```python
from build123d import *

# Parameters (mm, degrees)
F1_DEPTH = 63.5


with BuildPart() as f1:
    # F0 (on Front) → F1 (new body, symmetric)
    with BuildSketch(Plane.XZ):
        Polygon((60.325, 71.4502), (60.325, 61.5735440695), (83.1756805858, 61.5735440695), (83.1756805858, 42.8752), (111.125, 42.8752), (111.125, 71.4502), align=None)
        Polygon((22.225, 9.525), (-41.275, 9.525), (-41.275, -9.525), (41.275, -9.525), (41.275, 9.525), align=None)
        with BuildLine():
            add(Edge.make_bspline(
                [(-41.275, 9.525), (-1.6819942421, 36.6237502339), (37.9110115159, 63.7225004679), (59.4295399317, 61.5735440695)],
                knots=[0, 0, 0, 0, 0.658665778, 0.658665778, 0.658665778, 0.658665778], degree=3))
            Line((-41.275, 9.525), (22.225, 9.525))
            Line((22.225, 9.525), (22.225, 26.7230157708))
            ThreePointArc((22.225, 26.7230157708), (33.2738330873, 52.2119207798), (59.4295399317, 61.5735440695))
        make_face()
        with BuildLine():
            Line((83.1756805858, 42.8752), (82.928727027, 42.8752))
            add(Edge.make_bspline(
                [(82.928727027, 42.8752), (83.0110521067, 42.7579930507), (83.0933663462, 42.6407685601), (83.1756805858, 42.5235440695)],
                knots=[0.9955383683, 0.9955383683, 0.9955383683, 0.9955383683, 1, 1, 1, 1], degree=3))
            Line((83.1756805858, 42.5235440695), (83.1756805858, 42.8752))
        make_face()
        with BuildLine():
            Line((60.325, 61.5735440695), (59.4295399317, 61.5735440695))
            add(Edge.make_bspline(
                [(59.4295399317, 61.5735440695), (59.7315548679, 61.5433832278), (60.030009415, 61.5074610458), (60.325, 61.4659335595)],
                knots=[0.658665778, 0.658665778, 0.658665778, 0.658665778, 0.6679102253, 0.6679102253, 0.6679102253, 0.6679102253], degree=3))
            Line((60.325, 61.4659335595), (60.325, 61.5735440695))
        make_face()
        with BuildLine():
            Line((83.1756805858, 61.5735440695), (60.325, 61.5735440695))
            Line((60.325, 61.5735440695), (60.325, 61.4659335595))
            add(Edge.make_bspline(
                [(60.325, 61.4659335595), (70.7796236232, 59.9941773031), (76.8834021634, 51.4819828541), (82.928727027, 42.8752)],
                knots=[0.6679102253, 0.6679102253, 0.6679102253, 0.6679102253, 0.9955383683, 0.9955383683, 0.9955383683, 0.9955383683], degree=3))
            Line((82.928727027, 42.8752), (83.1756805858, 42.8752))
            Line((83.1756805858, 42.8752), (83.1756805858, 61.5735440695))
        make_face()
        with BuildLine():
            Line((22.225, 26.7230157708), (22.225, 9.525))
            Line((22.225, 9.525), (41.275, 9.525))
            Line((41.275, 9.525), (41.275, 26.7230157708))
            ThreePointArc((41.275, 26.7230157708), (46.4815063401, 38.4788172334), (58.6858810115, 42.5235440695))
            Line((58.6858810115, 42.5235440695), (83.1756805858, 42.5235440695))
            add(Edge.make_bspline(
                [(82.928727027, 42.8752), (83.0110521067, 42.7579930507), (83.0933663462, 42.6407685601), (83.1756805858, 42.5235440695)],
                knots=[0.9955383683, 0.9955383683, 0.9955383683, 0.9955383683, 1, 1, 1, 1], degree=3))
            Line((82.928727027, 42.8752), (60.325, 42.8752))
            Line((60.325, 42.8752), (60.325, 61.4659335595))
            add(Edge.make_bspline(
                [(59.4295399317, 61.5735440695), (59.7315548679, 61.5433832278), (60.030009415, 61.5074610458), (60.325, 61.4659335595)],
                knots=[0.658665778, 0.658665778, 0.658665778, 0.658665778, 0.6679102253, 0.6679102253, 0.6679102253, 0.6679102253], degree=3))
            ThreePointArc((59.4295399317, 61.5735440695), (33.2738330873, 52.2119207798), (22.225, 26.7230157708))
        make_face()
        with BuildLine():
            add(Edge.make_bspline(
                [(60.325, 61.4659335595), (70.7796236232, 59.9941773031), (76.8834021634, 51.4819828541), (82.928727027, 42.8752)],
                knots=[0.6679102253, 0.6679102253, 0.6679102253, 0.6679102253, 0.9955383683, 0.9955383683, 0.9955383683, 0.9955383683], degree=3))
            Line((60.325, 61.4659335595), (60.325, 42.8752))
            Line((60.325, 42.8752), (82.928727027, 42.8752))
        make_face()
    extrude(amount=F1_DEPTH, both=True)


solid = f1.part
```
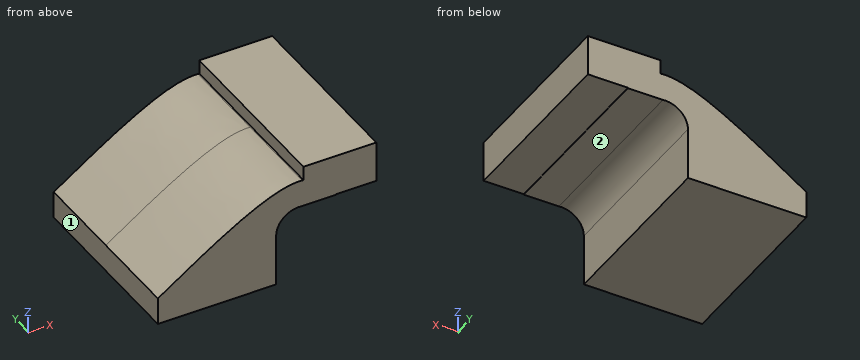
Geometry check sheet. Reference: the model listing, model coordinates, mm. Face numbers are marked on the shaded views. A direction names the side the tool comes from. Give positions to 0.01 mm unless a question says otherwise; leave off trailing zeros. Order: outer loops, then holes, each group sorted by start corner. A loop starts at its lowest first (then second) coordinate and runs counter-clockwise, first axis right, second up. Notation, with made-up numbers: (80, 26.25) -> (99, 26.25) arc R31 ccw to (99, 53.25) -> close; hole circle Ø1 at (33, 69.5). An arc over 180 degrees is marked (long way). Write each question's results on one line, items separated by ' | '. Start each with the question number.
(1) Sectioned sample at A-A (x = 91). Enter the section's corners in (y, z).
(2) Scan lines: line 1 (X direction, y = -34, z = 63.5) (3 decimals); line 2 (Z direction, x = 63, y = 25); line 3 (X direction, y = 45, z = -1.5) (3 decimals). Record each from-to range of solid material in increasing order.
(3) Sectioned sample at B-B (z = -3). Enter the section's corners in (x, y) (3 decimals).
(4) Access from +Z, -Z, +X, -X, +Y, -Y to the whole of each face (thin tool, end or side, straight path). Record for the marked faces 1 and 2.
(5) Gauge pin test, flat ends, axial feed: P1, Ø12, axis at x = 64, y = 0, coming from the -Z side; P2, Ø3, axis at y = -9.5, z = 64.5, coming from the -X side (3 decimals); P3, Ø4, axis at y = 47.5, z = 1.5, coming from the +X side (3 decimals). Record the tip position at first contact, or that the pin passes through.
Answer below:
1) outline: (-63.5, 42.88) -> (63.5, 42.88) -> (63.5, 71.45) -> (-63.5, 71.45) -> close
2) line 1: 60.325 to 111.125 | line 2: 42.52 to 71.45 | line 3: -41.275 to 41.275
3) outline: (-41.275, -63.5) -> (41.275, -63.5) -> (41.275, 63.5) -> (-41.275, 63.5) -> close
4) face 1: +Z, -Z, -X, +Y, -Y | face 2: -Z, +X, +Y, -Y
5) P1: z = 42.52 | P2: x = 60.325 | P3: x = 41.275
